Geometry: final body of the model. Coordinates: model frame, mm. Face numbers are marked on the shaded views. A direction names the side the tool comes from. Give positions to 0.01 mm unless a question says otherwise; leave off trailing zeros. Answer in a Markdown table with one row per item. Add a question column.
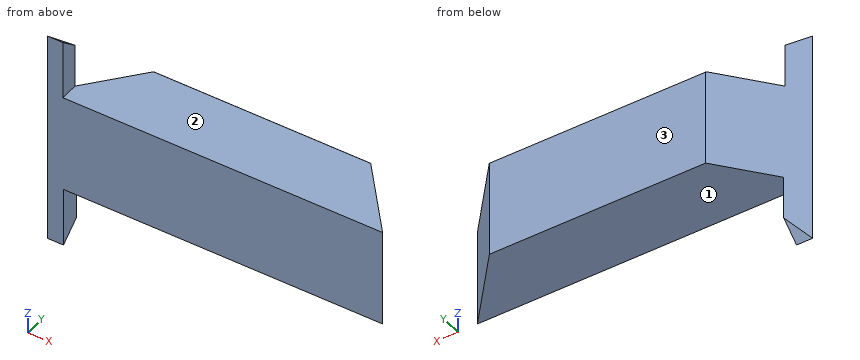
from build123d import *

# Parameters (mm, degrees)
F0_W     = 96.55572474
F0_H     = 43.4501469135
F1_DEPTH = 31.6610336304
F1_TAPER = -40
F2_W     = 167.0255586505
F2_H     = 38.3586026728
F2_W_2   = 162.8842428327
F2_H_2   = 31.8540707231
F3_DEPTH = 79.4451162219
F4_W     = 21.1209580302
F4_H     = 32.886043191
F5_DEPTH = 14.5127717406


with BuildPart() as f1:
    # F0 (on Front) → F1 (new body)
    with BuildSketch(Plane.XZ):
        Rectangle(F0_W, F0_H)
    extrude(amount=F1_DEPTH, taper=F1_TAPER)

    # F2 (on Front) → F3 (cut)
    with BuildSketch(Plane.XZ):
        with Locations((15.839908272, -40.9009512514)):
            Rectangle(F2_W, F2_H)
        with Locations((13.4780444205, 37.8784425557)):
            Rectangle(F2_W_2, F2_H_2)
    extrude(amount=F3_DEPTH, mode=Mode.SUBTRACT)

    # F4 (on Front) → F5 (cut)
    with BuildSketch(Plane.XZ):
        with Locations((-66.4090551436, 38.6971160769)):
            Rectangle(F4_W, F4_H)
    extrude(amount=F5_DEPTH, mode=Mode.SUBTRACT)


solid = f1.part
Q1. Line query: probe 1 along Z at (x, y) = (30, -5.5); probe 2 along Y at (x, z) = (55.5, 1); probe 3 along X at (y, z) = (-24.5, 36.5). Output: solid intervals per line, ascending. Write a range as from..to.
Q2. Access query for the marked faces 1, 2 and 3. Directions: +Z, -Z, +X, -X, +Y, -Y. A direction counts if a zero-diameter tool reaches every point of the face in a straight line with its end or side. Return the directions, or none.
Q3. Contact query for flat-ended pins moving along their axis: pin 1 Ø2.5 at (y, z) = (-27.5, -33) entering from +X; pin 2 Ø10 at (x, y) = (-1, -22) entering from +Z; pin 3 Ø8 at (x, y) = (22.5, -21.5) entering from -Z. Output: stop coordinate, or through.
Checks:
| question | item | result |
|---|---|---|
| 1 | probe 1 | -21.72..21.95 |
| 1 | probe 2 | -31.66..-8.61 |
| 1 | probe 3 | -68.84..-67.96 |
| 2 | face 1 | -Z, +X, +Y, -Y |
| 2 | face 2 | +Z, +X, +Y, -Y |
| 2 | face 3 | +Z, -Z, +X, -X, +Y |
| 3 | pin 1 | x = -67.67 |
| 3 | pin 2 | z = 21.95 |
| 3 | pin 3 | z = -21.72 |
